from build123d import *

# Parameters (mm, degrees)
SKETCH1_W           = 70
SKETCH1_H           = 30
SKETCH1_R           = 10.5
BOSS_EXTRUDE1_DEPTH = 4
SKETCH3_W           = 8.150987667
SKETCH3_H           = 10.43538234
SKETCH3_W_2         = 6.820916115
SKETCH3_H_2         = 20
BOSS_EXTRUDE2_DEPTH = 17
SKETCH4_R           = 1
CUT_EXTRUDE1_DEPTH  = 17
BOSS_EXTRUDE4_DEPTH = 3
BOSS_EXTRUDE5_DEPTH = 20
SKETCH10_R          = 2.75
CUT_EXTRUDE2_DEPTH  = 47.25


with BuildPart() as part:
    # Sketch1 → Boss-Extrude1 (new body)
    with BuildSketch(Plane.XY):
        with Locations((35, -15)):
            Rectangle(SKETCH1_W, SKETCH1_H)
        with Locations((35, -15)):
            Circle(SKETCH1_R, mode=Mode.SUBTRACT)
    extrude(amount=BOSS_EXTRUDE1_DEPTH)

    # Sketch3 → Boss-Extrude2 (add)
    with BuildSketch(Plane(origin=(0, 0, 0), x_dir=(-1, 0, 0), z_dir=(0, 0, -1))):
        with Locations((-58.424506167, -14.156074174)):
            Rectangle(SKETCH3_W, SKETCH3_H)
        with Locations((-10.910458058, -15)):
            Rectangle(SKETCH3_W_2, SKETCH3_H_2)
    extrude(amount=BOSS_EXTRUDE2_DEPTH)

    # Sketch4 → Cut-Extrude1 (cut)
    with BuildSketch(Plane(origin=(0, 0, -17), x_dir=(-1, 0, 0), z_dir=(0, 0, -1))):
        with Locations((-58.5, -14.289099526)):
            Circle(SKETCH4_R)
        with Locations((-11.5, -7)):
            Circle(SKETCH4_R)
        with Locations((-11.5, -23)):
            Circle(SKETCH4_R)
    extrude(amount=-CUT_EXTRUDE1_DEPTH, mode=Mode.SUBTRACT)

    # Sketch7 → Boss-Extrude4 (add)
    with BuildSketch(Plane(origin=(0, 0, 0), x_dir=(1, 0, 0), z_dir=(0, 1, 0))):
        Polygon((-4.630368757, -4), (65.882216562, -22.893790292), (73.129149825, 4.152132844), (2.616564506, 23.045923136), align=None)
    extrude(amount=BOSS_EXTRUDE4_DEPTH)

    # Sketch9 → Boss-Extrude5 (add)
    with BuildSketch(Plane(origin=(0, 3, 0), x_dir=(1, 0, 0), z_dir=(0, 1, 0))):
        Polygon((-4.630368757, -4), (65.882216562, -22.893790292), (66.875377983, -19.18726141), (-3.595092577, -0.136296695), align=None)
        Polygon((2.616564506, 23.045923136), (1.581288325, 19.182219831), (72.093873644, 0.288429538), (73.129149825, 4.152132844), align=None)
    extrude(amount=BOSS_EXTRUDE5_DEPTH)

    # Sketch10 → Cut-Extrude2 (cut, through all)
    with BuildSketch(Plane(origin=(5.936757371, 0, -22.156280139), x_dir=(-0.965925826, 0, -0.258819045), z_dir=(0.258819045, 0, -0.965925826))):
        with Locations((-53.953749554, 11.5)):
            Circle(SKETCH10_R)
        with Locations((-12.488324975, 11.5)):
            Circle(SKETCH10_R)
    extrude(amount=-CUT_EXTRUDE2_DEPTH, mode=Mode.SUBTRACT)


solid = part.part
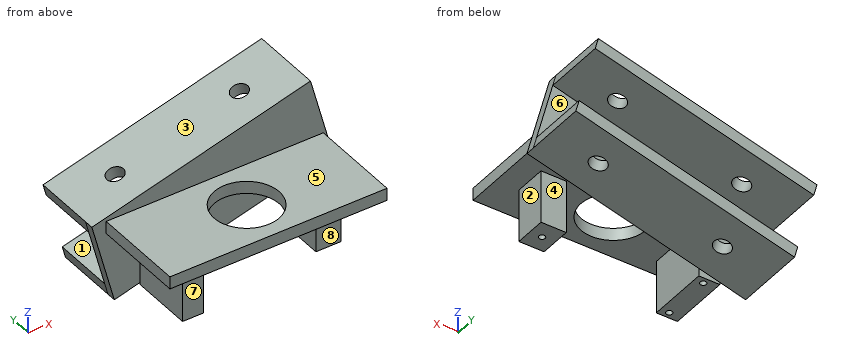
The listing builds one solid part. Answer for the finished solid, in the listing's coordinates (mm). Face numbers are marked on the shaded views. A direction names the side the tool comes from. Coordinates: 2 decimals unless noted, no trailing zeros. Loops run counter-clockwise (first coordinate to the right, second up) from the corner with the lowest first, then second, coordinate; pieces in that order, holes last.
1) Find section D-D on z = 2. Write down the section's boundary in (x, y).
2) A tool of negligible diameter and unlimited length cuts with its end or side. For the marked faces 4, 5, 6, 7 and 8, from which of +Z, -Z, +X, -X, +Y, -Y can it reach the whole face along a straight path? Write none if from no direction.
3) Determine the mould class of the marked faces 1, 2 and 3 for opening direction Z: pulls with the +Z half, pulls with the -Z half, needs draft (parallel to the pull), parting line crosses it, or undercut.
4) Find section B-B on y = 16. Write down the section's boundary in (x, z), then the cut area to 3 significant figures.
5) Find section C-C on x = 35. Write down the section's boundary in (y, z), then the cut area to 3 significant figures.
6) Find section A-A on z = -11. Write down the section's boundary in (x, y).
7) Find the intervals of material crossed by L1, parallel to Y at x = 11.5, z = -7.75; L2, parallel to Y at x = 11, z = -7; L3, parallel to X at y = -11, z = -14.5, in increasing order.
8) Flat-ended cylindrical pins translate along their axes: pin 1 Ø4.5 at (y, z) = (-20.5, 1) entering from +X; pin 2 Ø18.5 at (y, z) = (-12.5, -12) entering from -X; pin 3 Ø3 at (x, y) = (11.5, -23) entering from -Z. Find the tip coordinate at first contact, or state that the pin passes through.
Values:
1. outline: (-4.09, 0) - (0, 0) - (0, -30) - (70, -30) - (70, 0) - (71.48, 0) - (71.48, 3) - (3.3, 3) - (3.3, 23) - (-4.09, 23) - close; hole circle Ø21 at (35, -15)
2. face 4: -Z, +X
2. face 5: +Z, +X, -X, -Y
2. face 6: +Y
2. face 7: -Z, +X, -X, -Y
2. face 8: -Z, +X, -Y
3. face 1: undercut
3. face 2: needs draft
3. face 3: pulls with the +Z half
4. outline: (-4.63, 4) - (-3.6, 0.14) - (66.88, 19.19) - (65.88, 22.89) - close; (1.58, -19.18) - (2.62, -23.05) - (73.13, -4.15) - (72.09, -0.29) - close
4. area: 578 mm2
5. outline: (-30, 0) - (-25.5, 0) - (-25.5, 4) - (-30, 4) - close; (-4.5, 0) - (0, 0) - (0, -14.37) - (23, -14.37) - (23, -10.23) - (3, -10.23) - (3, 10.57) - (23, 10.57) - (23, 14.62) - (0, 14.62) - (0, 4) - (-4.5, 4) - close
5. area: 287 mm2
6. outline: (-0.61, 0) - (47.57, 0) - (47.57, 23) - (32.12, 23) - (32.12, 3) - (-0.61, 3) - close; (7.5, -25) - (14.32, -25) - (14.32, -5) - (7.5, -5) - close; (54.35, -19.37) - (62.5, -19.37) - (62.5, -8.94) - (54.35, -8.94) - close; hole circle Ø2 at (11.5, -23); hole circle Ø2 at (11.5, -7); hole circle Ø2 at (58.5, -14.29)
7. L1: y = -25 to -24, -22 to -8, -6 to -5, 0 to 3
7. L2: y = -25 to -23.87, -22.13 to -7.87, -6.13 to -5, 0 to 3
7. L3: x = 7.5 to 14.32, 54.35 to 62.5
8. pin 1: stops at x = 70
8. pin 2: stops at x = 7.5
8. pin 3: stops at z = -17
